Input: part model. Units: mm. Frame: model coordinates. Face numbers are marked on the shaded views. A direction names the side the tool comes from. Coordinates: 2 decimals unless noted, no trailing zeros. Write each loop counter-clockwise with the first axis right and the second up, starting at its lowest first coordinate (ties: lowest second). Pieces come first, ordered by that corner, then holes. Notation, with made-up numbers: (-40, -4.75) - (-13, -4.75) arc R23 cw to (-13, 32.25) - close; hole circle Ø9 at (-23, 57). An arc over 180 degrees is marked (long way). One line per question, with ' | ' between items. Start each with the question number.
1) Draft query along Y for the marked faces 3, 4 and 5. Return one class per face: released by +Y, released by -Y, zero draft, split by the parting line, or undercut.
2) First-contact query: P1, Ø2.5, axis at y = 4, z = 3.5, coming from the -X side; P2, Ø2, axis at x = 5.5, z = 5, coming from the -Y side; P3, Ø1.9, axis at x = 1, z = 3.5, coming from the -Y side; P4, Ø0.5, axis at y = 0.5, z = 3.5, coming from the +X side. Flat tips, straight axial feed; report the tip coordinate or a pass-through.
3) Section query D-D on z = 2. Return loops of the section in (x, y), and give its area (3 significant figures).
4) Reachability of the marked faces 1 and 2 from +Z, -Z, +X, -X, +Y, -Y: full face, straight path, thin tool, end or side. Return the list, or none.
5) Section query B-B on y = 6.5. Return loops of the section in (x, z).
6) Section query A-A on z = 4.5. Return loops of the section in (x, y), and give its area (3 significant figures).
7) Line query: line 1 (Y direction, x = 0.5, z = 2.5); line 2 (Y direction, x = 9, z = 2); line 3 (Y direction, x = 2, z = 3.5). Output: solid intervals per line, ascending.
8) Section query C-C on x = 8. Return loops of the section in (y, z).
```python
from build123d import *

# Parameters (mm, degrees)
SKETCH_W        = 10
SKETCH_H        = 10
PAD_DEPTH       = 0.8
SKETCH001_W     = 6
SKETCH001_H     = 5
PAD001_DEPTH    = 6
CHAMFER_SIZE    = 5
CHAMFER001_SIZE = 0.7


with BuildPart() as part:
    # Sketch → Pad (new body)
    with BuildSketch(Plane.XY):
        with Locations((5, 5)):
            Rectangle(SKETCH_W, SKETCH_H)
    extrude(amount=PAD_DEPTH)

    # Sketch001 (on Face6 of Pad) → Pad001 (join)
    with BuildSketch(Plane.XY.offset(0.8)):
        with Locations((7, 5)):
            Rectangle(SKETCH001_W, SKETCH001_H)
        Polygon((0, 0.8), (0, 2.6), (0.8, 2.6), (0.8, 1.6), (2.4, 1.6), (2.4, 0.8), align=None)
        Polygon((0, 7.403696), (0, 9.203696), (2.399997, 9.2), (2.399997, 8.4), (0.8, 8.402464), (0.8, 7.402464), align=None)
    extrude(amount=PAD001_DEPTH)

    # Chamfer
    chamfer_edges = [part.edges().sort_by_distance(p)[0] for p in [
        (10, 5, 6.8),
    ]]
    chamfer(chamfer_edges, length=CHAMFER_SIZE)

    # Chamfer001
    chamfer001_edges = [part.edges().sort_by_distance(p)[0] for p in [
        (1.2, 0.8, 0.8),
        (1.199999, 9.201848, 0.8),
    ]]
    chamfer(chamfer001_edges, length=CHAMFER001_SIZE)


solid = part.part
```
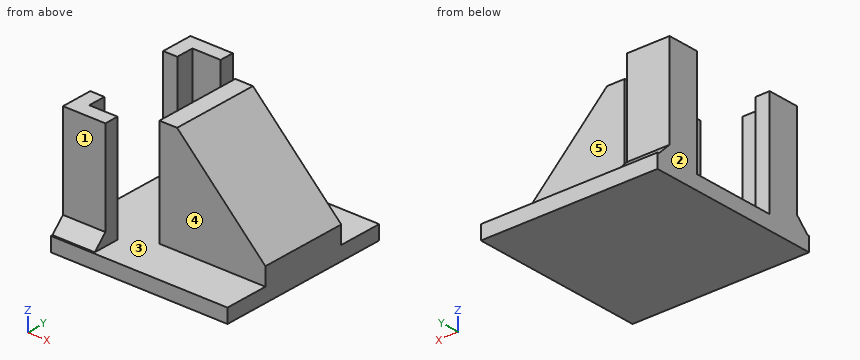
Answer key:
1) face 3: undercut | face 4: released by -Y | face 5: released by +Y
2) P1: x = 4 | P2: y = 2.5 | P3: y = 0.8 | P4: through
3) outline: (0, 0.8) - (2.4, 0.8) - (2.4, 1.6) - (0.8, 1.6) - (0.8, 2.6) - (0, 2.6) - close; (0, 7.4) - (0.8, 7.4) - (0.8, 8.4) - (2.4, 8.4) - (2.4, 9.2) - (0, 9.2) - close; (4, 2.5) - (9.8, 2.5) - (9.8, 7.5) - (4, 7.5) - close | area: 34.4 mm²
4) face 1: +Z, +X, -X, -Y | face 2: +Z, -Z, -X, +Y, -Y
5) outline: (0, 0) - (10, 0) - (10, 1.8) - (5, 6.8) - (4, 6.8) - (4, 0.8) - (0, 0.8) - close
6) outline: (0, 0.8) - (2.4, 0.8) - (2.4, 1.6) - (0.8, 1.6) - (0.8, 2.6) - (0, 2.6) - close; (0, 7.4) - (0.8, 7.4) - (0.8, 8.4) - (2.4, 8.4) - (2.4, 9.2) - (0, 9.2) - close; (4, 2.5) - (7.3, 2.5) - (7.3, 7.5) - (4, 7.5) - close | area: 21.9 mm²
7) line 1: 0.8 to 2.6, 7.4 to 9.2 | line 2: 2.5 to 7.5 | line 3: 0.8 to 1.6, 8.4 to 9.2
8) outline: (0, 0) - (10, 0) - (10, 0.8) - (7.5, 0.8) - (7.5, 3.8) - (2.5, 3.8) - (2.5, 0.8) - (0, 0.8) - close
